Geometry: final body of the model. Coordinates: model frame, mm. A direction names the side the tool comes from. Give positions to 0.01 mm unless a question says otherwise; leave off trailing zeros. Loops run counter-clockwise (first coordinate to the right, second up) from the corner with the lowest first, then second, coordinate; pieces in that order, holes last.
1. Draft query along X for faces 3 (the face through (10, 0, 12)), 4 (the face through (0, -1, 0)), 5 (the face through (-8.2, -10, 7.6)). Return one class per face: +X half, -X half, draft (parallel to the pull), parting line (faces both ways), or undercut.
2. First-contact query: P1, Ø2, axis at x = -2.5, z = 18.5, coming from the -Y side; P2, Ø2, axis at x = 3, y = 3.5, coming from the +Z side. Flat tips, straight axial feed; report the tip coordinate or a pass-through.
3. Section A-A, the plane z = 15. Output: boundary loops of the cut face in (x, y).
4. Section B-B, the plane x = 2.5. Output: boundary loops of the cut face in (y, z), then the cut area to 3 significant figures.
5. Material intervals for line 1 along X through (y, z) = (1, 17); line 2 along Y through (x, z) = (2.75, 22.5); line 3 along Z through (x, y) = (3, 6.75), sorted ascending.
6. Access query for faces 1 (the face through (0, 8, 12)), 2 (the face through (-10, 0, 12)). Directions: +Z, -Z, +X, -X, +Y, -Y. A direction counts if a zero-diameter tool reaches every point of the face in a straight line with its end or side. Return the directions, or none.
7. Section C-C, the plane y = 6.75. Output: boundary loops of the cut face in (x, z), then the cut area to 3 significant figures.
from build123d import *

# Parameters (mm, degrees)
F1_DEPTH = 25
F0_W     = 16
F0_H     = 18
F2_DEPTH = 2


with BuildPart() as f1:
    # F0 (on Top) → F1 (new body)
    with BuildSketch(Plane.XY):
        Polygon((10, 10), (-10, 10), (-10, -10), (-8, -10), (-8, 8), (8, 8), (8, -10), (10, -10), align=None)
    extrude(amount=F1_DEPTH)

    # F0 (on Top) → F2 (join)
    with BuildSketch(Plane.XY):
        Polygon((10, 10), (-10, 10), (-10, -10), (-8, -10), (-8, 8), (8, 8), (8, -10), (10, -10), align=None)
        with Locations((0, -1)):
            Rectangle(F0_W, F0_H)
    extrude(amount=-F2_DEPTH)


solid = f1.part
Answers below:
1. face 3: +X half
1. face 4: undercut
1. face 5: draft
2. P1: stops at y = 8
2. P2: stops at z = 0
3. outline: (-10, -10) - (-8, -10) - (-8, 8) - (8, 8) - (8, -10) - (10, -10) - (10, 10) - (-10, 10) - close
4. outline: (-10, -2) - (10, -2) - (10, 25) - (8, 25) - (8, 0) - (-10, 0) - close
4. area: 90.0 mm2
5. line 1: x = -10 to -8, 8 to 10
5. line 2: y = 8 to 10
5. line 3: z = -2 to 0
6. face 1: +Z, -Y
6. face 2: +Z, -Z, -X, +Y, -Y
7. outline: (-10, -2) - (10, -2) - (10, 25) - (8, 25) - (8, 0) - (-8, 0) - (-8, 25) - (-10, 25) - close
7. area: 140 mm2
